Autodesk Inventor part; units mm, degrees
ref_plane "YZ Plane" through (0, 0, 0) normal (1, 0, 0) x (0, 1, 0)
ref_plane "XZ Plane" through (0, 0, 0) normal (0, 1, 0) x (-1, 0, 0)
ref_plane "XY Plane" through (0, 0, 0) normal (0, 0, 1) x (1, 0, 0)
sketch "Sketch1" plane through (0, 0, 0) normal (0, 0, 1) x (1, 0, 0)
  line L0 (0, 0) -> (-25.4, 0)
  line L1 (-25.4, 0) -> (-25.4, 25.4)
  line L2 (-25.4, 25.4) -> (0, 25.4)
  line L3 (0, 25.4) -> (0, 0)
  line L4 (-3.175, 22.225) -> (-22.225, 22.225)
  line L5 (-22.225, 22.225) -> (-22.225, 3.175)
  line L6 (-22.225, 3.175) -> (-3.175, 3.175)
  line L7 (-3.175, 3.175) -> (-3.175, 22.225)
  dimension "d0" = 25.4
  dimension "d1" = 25.4
  dimension "d2" = 3.175
extrude "Extrusion1" add sketch "Sketch1" along normal blind 86.36
sketch "Sketch2" plane through (-25.4, 25.4, 0) normal (0, 1, 0) x (1, 0, 0)
  line L0 (0, 0) -> (25.4, 0)
  line L1 (25.4, 0) -> (25.4, -86.36)
  line L2 (12.7, 0) -> (12.7, -12.7)
  circle A0 centre (12.7, -12.7) radius 3.3782
  dimension "d5" = 12.7
  dimension "d6" = 6.7564
extrude "Extrusion2" cut sketch "Sketch2" against normal blind 86.36
pattern_linear "Rectangular Pattern1" count 3 spacing 25.4 along (0, 0, 1) of "Extrusion2"
properties part number "corner bumper mount" material "Aluminum 6061"
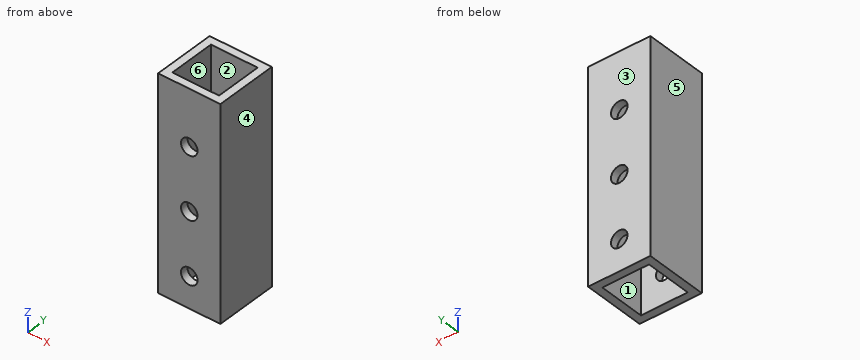
The listing builds one solid part. Answer for the finished solid, in the listing's coordinates (mm). Face numbers are marked on the shaded views. A direction names the side the tool comes from. Coordinates: 2 decimals unless noted, no trailing zeros. Write each loop counter-clockwise with the first axis right and the second up, starting at its lowest first coordinate (ties: lowest second). Pieces come first, ordered by that corner, then holes. Notation, with made-up numbers: M -22.5,-29.75 L -11.5,-29.75 A17 cw -11.5,-23.75 Z; hole C -34,46.5 d9. An arc over 180 degrees is marked long. Use one line per item in the form item = value.
Item 1: The mould has two halves that part along X. Classify the marked faces 1, 2, 3 and 4: released by +X, released by -X, zero draft, split by the parting line, or undercut.
Model answer:
face_1 = undercut
face_2 = undercut
face_3 = zero draft
face_4 = released by +X
Item 2: Find section C-C, the plane x = -12.7. Give the number of separate pieces and of enclosed holes in the cut face, plus the area to 3 significant figures.
Model answer:
separate_pieces = 8
enclosed_holes = 0
area = 420 mm2
Item 3: Find section D-D, the plane z = 75.5. Give the vertices of the cut face in (x, y) (3 decimals).
Model answer:
outline = M -25.4,0 L 0,0 L 0,25.4 L -25.4,25.4 Z; hole M -22.225,3.175 L -3.175,3.175 L -3.175,22.225 L -22.225,22.225 Z
Item 4: Find the intervals of material crossed by probe 1 along Z at (x, y) = (-12.7, 1.8); probe 2 along X at (y, z) = (3.75, 46) (3 decimals); probe 3 along Y at (x, z) = (-21, 64) (3 decimals), in increasing order.
Model answer:
probe_1 = 0 to 9.32, 16.08 to 34.72, 41.48 to 60.12, 66.88 to 86.36
probe_2 = -25.4 to -22.225, -3.175 to 0
probe_3 = 0 to 3.175, 22.225 to 25.4
Item 5: Find section A-A, the plane z = 12.7. Give the vertices of the cut face in (x, y) (3 decimals), plus the area to 3 significant figures.
Model answer:
outline = M -25.4,0 L -16.078,0 L -16.078,3.175 L -22.225,3.175 L -22.225,22.225 L -16.078,22.225 L -16.078,25.4 L -25.4,25.4 Z; M -9.322,0 L 0,0 L 0,25.4 L -9.322,25.4 L -9.322,22.225 L -3.175,22.225 L -3.175,3.175 L -9.322,3.175 Z
area = 239 mm2
Item 6: Find section B-B, the plane y = 17.75. Give the vertices of the cut face in (x, z) (3 decimals).
Model answer:
outline = M -25.4,0 L -22.225,0 L -22.225,86.36 L -25.4,86.36 Z; M -3.175,0 L 0,0 L 0,86.36 L -3.175,86.36 Z
Item 7: For the marked faces 5 and 6, determine the directions among +Z, -Z, +X, -X, +Y, -Y from which every point of the face is accessible in a straight line to the end or side of a thin tool.
Model answer:
face_5 = +Z, -Z, -X, +Y, -Y
face_6 = +Z, -Z
